from build123d import *

# Parameters (mm, degrees)
SKETCH1_W                                    = 220
SKETCH1_H                                    = 220
BOSS_EXTRUDE1_DEPTH                          = 3
FILLET1_R                                    = 5
CSK_FOR_M4_COUNTERSUNK_FLAT_HEAD_SCR_2_COUNT = 2
CSK_FOR_M4_COUNTERSUNK_FLAT_HEAD_SCR_2_PITCH = 209
CSK_FOR_M4_COUNTERSUNK_FLAT_HEAD_SCR_3_COUNT = 2
CSK_FOR_M4_COUNTERSUNK_FLAT_HEAD_SCR_3_PITCH = 209
CSK_FOR_M4_COUNTERSUNK_FLAT_HEAD_SCR_4_COUNT = 2
CSK_FOR_M4_COUNTERSUNK_FLAT_HEAD_SCR_4_PITCH = 295.570634536


with BuildPart() as part:
    # Sketch1 → Boss-Extrude1 (new body)
    with BuildSketch(Plane(origin=(0, 0, 0), x_dir=(1, 0, 0), z_dir=(0, 1, 0))):
        Rectangle(SKETCH1_W, SKETCH1_H)
    extrude(amount=BOSS_EXTRUDE1_DEPTH)

    # Fillet1
    fillet1_edges = [part.edges().sort_by_distance(p)[0] for p in [
        (110, 1.5, 110),
        (-110, 1.5, 110),
        (-110, 1.5, -110),
        (110, 1.5, -110),
    ]]
    fillet(fillet1_edges, radius=FILLET1_R)

    # Sketch4 → CSK for M4 Countersunk Flat Head Screw1 (revolve, cut)
    with BuildSketch(Plane(origin=(-104.5, 3, -104.5), x_dir=(0, 0, 1), z_dir=(1, 0, 0))):
        Polygon((0, 0), (0, 3), (2.25, 3), (2.25, 2.45), (4.7, 0), align=None)
    csk_for_m4_countersunk_flat_head_screw1 = revolve(axis=Axis((-104.5, 9.35, -104.5), (0, -1, 0)), mode=Mode.SUBTRACT)

    # CSK for M4 Countersunk Flat Head Scr 2: CSK for M4 Countersunk Flat Head Screw1 ×2
    with Locations(*[(i * CSK_FOR_M4_COUNTERSUNK_FLAT_HEAD_SCR_2_PITCH, 0, 0) for i in range(1, CSK_FOR_M4_COUNTERSUNK_FLAT_HEAD_SCR_2_COUNT)]):
        add(csk_for_m4_countersunk_flat_head_screw1, mode=Mode.SUBTRACT)

    # CSK for M4 Countersunk Flat Head Scr 3: CSK for M4 Countersunk Flat Head Screw1 ×2
    with Locations(*[(0, 0, i * CSK_FOR_M4_COUNTERSUNK_FLAT_HEAD_SCR_3_PITCH) for i in range(1, CSK_FOR_M4_COUNTERSUNK_FLAT_HEAD_SCR_3_COUNT)]):
        add(csk_for_m4_countersunk_flat_head_screw1, mode=Mode.SUBTRACT)

    # CSK for M4 Countersunk Flat Head Scr 4: CSK for M4 Countersunk Flat Head Screw1 ×2
    with Locations(*[Vector(0.707106781, 0, 0.707106781) * (i * CSK_FOR_M4_COUNTERSUNK_FLAT_HEAD_SCR_4_PITCH) for i in range(1, CSK_FOR_M4_COUNTERSUNK_FLAT_HEAD_SCR_4_COUNT)]):
        add(csk_for_m4_countersunk_flat_head_screw1, mode=Mode.SUBTRACT)


solid = part.part
Build history of the part. All positions in model axes, mm. Coordinates: 2 decimals unless noted, no trailing zeros.
(1) Drill centre line: line 1 (Z direction, x = 104.5, y = 0.3). Where is it in solid material? Low to high.
(2) Mould opens along Z. For faces 1 (the cylindrical face through (109, 2, -108)), 2 (the flat face through (-2, 3, -2)), 3 (the cylindrical face through (108, 2, 109)), 4 (the conical face through (105.962, 0.703, -106.407)) say: pulls with the +Z half, pulls with the -Z half, needs draft (parallel to the pull), parting line crosses it, or undercut.
(3) Pin check, flat tip, straight feed: pin 1 Ø6 at (x, z) = (104.5, -104.5) entering from +Y. Stop position of the tip, or through.
Working result:
1. line 1: z = -110 to -106.75, -102.25 to 102.25, 106.75 to 110
2. face 1: pulls with the -Z half
2. face 2: needs draft
2. face 3: pulls with the +Z half
2. face 4: undercut
3. pin 1: stops at y = 1.3
